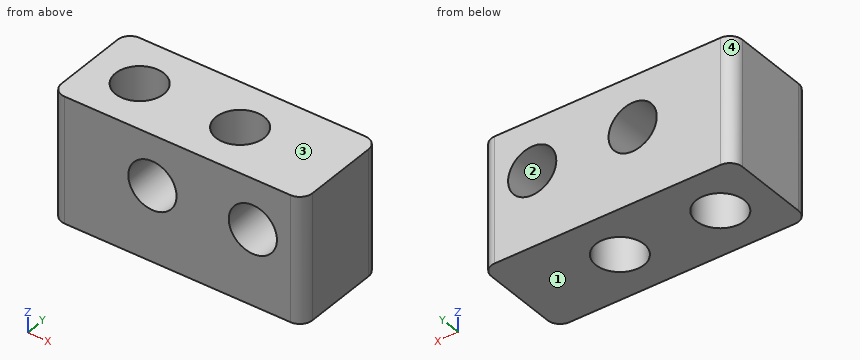
Autodesk Inventor part; units mm, degrees
ref_plane "YZ Plane" through (0, 0, 0) normal (1, 0, 0) x (0, 1, 0)
ref_plane "XZ Plane" through (0, 0, 0) normal (0, 1, 0) x (-1, 0, 0)
ref_plane "XY Plane" through (0, 0, 0) normal (0, 0, 1) x (1, 0, 0)
sketch "Sketch1" plane through (0, 0, 0) normal (0, 0, 1) x (1, 0, 0)
  line L0 (15.875, -6.35) -> (-15.875, -6.35)
  line L1 (-15.875, -6.35) -> (-15.875, 6.35)
  line L2 (-15.875, 6.35) -> (15.875, 6.35)
  line L3 (15.875, 6.35) -> (15.875, -6.35)
  line L4 (15.875, -6.35) -> (-15.875, 6.35) construction
  line L5 (-15.875, -6.35) -> (15.875, 6.35) construction
  point P0 (0, 0)
  dimension "d0" = 31.75
  dimension "d1" = 12.7
extrude "Extrusion1" add sketch "Sketch1" along normal blind 15.875
sketch "Sketch2" plane through (0, 0, 0) normal (0, 0, -1) x (-1, 0, 0)
  line L0 (15.875, 6.35) -> (15.875, -6.35)
  point P0 (0, 0)
  point P1 (9.525, 0)
  point P2 (-3.175, 0)
  dimension "d4" = 12.7
  dimension "d5" = 6.35
hole "Hole1" at (-9.525, 0, 0) at (3.175, 0, 0) direction (0, 0, 1) diameter 6.096 end through all
sketch "Sketch3" plane through (-15.875, -6.35, 0) normal (0, -1, 0) x (1, 0, 0)
  line L0 (0, 0) -> (0, 15.875)
  line L1 (0, 0) -> (31.75, 0)
  point P0 (15.875, 0)
  point P1 (12.7, 9.525)
  point P2 (25.4, 9.525)
  dimension "d13" = 12.7
  dimension "d14" = 12.7
  dimension "d15" = 9.525
hole "Hole2" at (-3.175, -6.35, 9.525) at (9.525, -6.35, 9.525) direction (0, 1, 0) diameter 6.096 end through all
fillet "Fillet1" radius 1.5875 4 edges at (-15.875, -6.35, 7.9375) (-15.875, 6.35, 7.9375) (15.875, -6.35, 7.9375) (15.875, 6.35, 7.9375)
properties part number "3DPRINT,LEFT,NUT-BLOCK" material "Nylon 6/6"
Can you work these out from the model? Positions are in its coordinate system, mm. Face numbers are marked on the shaded views. Round coordinates to 2 decimals unless told otherwise and drop trailing zeros. Loops run counter-clockwise (first coordinate to the right, second up) from the corner with the lowest first, then second, coordinate; pieces in that order, holes last. Notation, with made-up numbers: (85, 32.5) - (93, 32.5) arc R35 cw to (93, 66.5) - close; hole circle Ø9 at (83.5, -34). An arc over 180 degrees is marked (long way). Write item = value, one per line. Start each with the question number.
(1) If I drill on probe 1 along X at (y, z) = (0, 4) (3 decimals); probe 2 along X at (y, z) = (5.25, 12.25); probe 3 along Y at (x, z) = (3, 1.25), over which ranges is the centre line in solid material (lowest first)? Write a range as [from, to].
(2) For P1, Ø4, axis at x = -3, z = 9, coming from the -Y side, with a flat end and sliding along its axis, tell me the tip position at first contact or that it passes through.
(3) If we section it at A-A (z = 7): Give the number of separate pieces and of enclosed holes in the cut face, and give its area (3 significant figures).
(4) If we section it at C-C (x = -7): Please give me the cut outline in (y, z) (3 decimals), and give its area (3 significant figures).
(5) If we mould it in two halves opening along Z, with no side actions, what happens to the marked faces 1, 2, 3 and 4? For each: released by +Z, released by -Z, zero draft, split by the parting line, or undercut.
(6) If we section it at B-B (y = 0): Please give me the cut outline in (x, z) (3 decimals), and give its area (3 significant figures).
Ans:
q1.probe_1 = [-15.875, -12.573], [-6.477, 0.127], [6.223, 15.875]
q1.probe_2 = [-15.8, -4.54], [-1.81, 8.16], [10.89, 15.8]
q1.probe_3 = [-6.35, -3.04], [3.04, 6.35]
q2.P1 = through
q3.separate_pieces = 3
q3.enclosed_holes = 2
q3.area = 256 mm²
q4.outline = (-6.35, 0) - (-1.707, 0) - (-1.707, 15.875) - (-6.35, 15.875) - close; (1.707, 0) - (6.35, 0) - (6.35, 15.875) - (1.707, 15.875) - close
q4.area = 147 mm²
q5.face_1 = released by -Z
q5.face_2 = undercut
q5.face_3 = released by +Z
q5.face_4 = zero draft
q6.outline = (-15.875, 0) - (-12.573, 0) - (-12.573, 15.875) - (-15.875, 15.875) - close; (-6.477, 0) - (0.127, 0) - (0.127, 15.875) - (-6.477, 15.875) - close; (6.223, 0) - (15.875, 0) - (15.875, 15.875) - (6.223, 15.875) - close; hole circle Ø6.096 at (-3.175, 9.525); hole circle Ø6.096 at (9.525, 9.525)
q6.area = 252 mm²
